Part print with two shaded views. Sizes in mm from the minimum x, y, z corner. A direction names the side the tool comes from. Give positions to 0.01 mm unless a question says otherwise; leave off trailing zeros. Write each loop counter-clockwise with the first axis right and the second up, starting at its lowest first coordinate (ties: lowest second). Pieces come first, ordered by that corner, then holes. Notation, with made-up numbers: M 88,-13 L 143,-13 A25 ccw 143,14 Z; hole C -25,-21 d2. An arc over 180 degrees is marked long. Return JSON: item names as keys, results as strings. Group by question number.
Q1. Pull direction Y, two halves, no side cores. Call the marked faces 3, 4 and 5: +Y half, -Y half, draft (parallel to the pull), parting line (faces both ways), or undercut.
Q2. Tool access for the marked faces 1 and 2: list every direction of +Z, -Z, +X, -X, +Y, -Y with a clear straight run to the whole face (end or side of a thin tool).
Q3. Wall check: probe 1 along Y at (x, z) = (6, 11) (1 decimal); probe 2 along Y at (x, z) = (9.5, 18.5) (1 decimal); probe 3 along Z at (x, y) = (16.5, 10.5). Give the ranges that are in metal, low to high.
Q4. Band-saw the part on A-A, the plane z = 16. Give the cut face in (x, y) (1 decimal).
Q5. Band-saw the part on C-C, the plane y = 11. Give the cut face in (x, z).
Q6. Flat gauge pins, fed straight in: pin 1 Ø0.9 at (x, z) = (17.52, 3.17) entering from +Y; pin 2 Ø1 at (x, y) = (11.5, 12) entering from -Z; pin 3 Ø1.5 at (x, y) = (19, 16) entering from -Z. Where does each tip first touch, or does it go through?
Q7. Band-saw the part on B-B, the plane x = 9. Give the cut face in (y, z) (1 decimal).
Q8. Band-saw the part on D-D, the plane x = 13. Give the cut face in (y, z) (1 decimal).
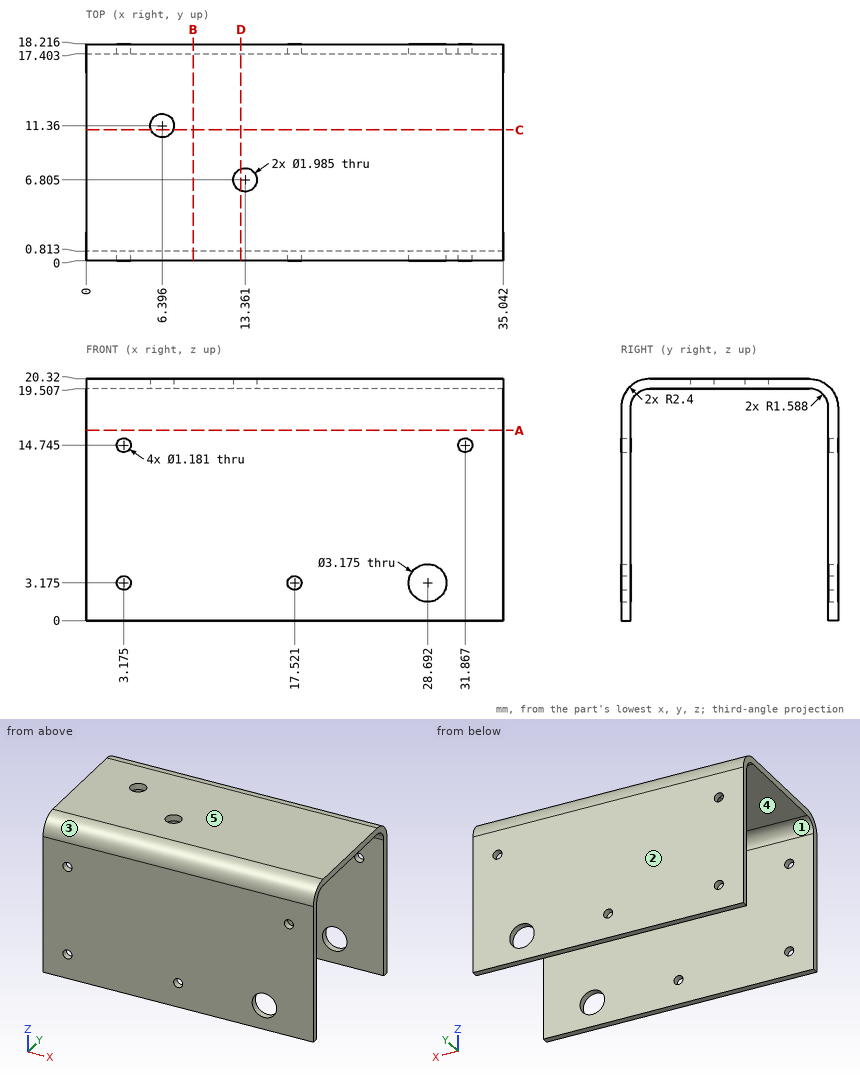
From the geometry:
{
 "1": {"face 3": "-Y half", "face 4": "undercut", "face 5": "draft"},
 "2": {"face 1": "-Z, +X, -X", "face 2": "+Z, -Z, +X, -X, +Y"},
 "3": {"probe 1": "y = 0 to 0.8, 17.4 to 18.2", "probe 2": "y = 0.1 to 0.9, 17.3 to 18.1", "probe 3": "z = 19.51 to 20.32"},
 "4": {"outline": "M 0,0 L 35,0 L 35,0.8 L 0,0.8 Z; M 0,17.4 L 35,17.4 L 35,18.2 L 0,18.2 Z"},
 "5": {"outline": "M 0,19.51 L 5.47,19.51 L 5.47,20.32 L 0,20.32 Z; M 7.32,19.51 L 35.04,19.51 L 35.04,20.32 L 7.32,20.32 Z"},
 "6": {"pin 1": "passes through", "pin 2": "stops at z = 19.51", "pin 3": "stops at z = 19.2"},
 "7": {"outline": "M 0,0 L 0.8,0 L 0.8,17.9 A1.6 cw 2.4,19.5 L 15.8,19.5 A1.6 cw 17.4,17.9 L 17.4,0 L 18.2,0 L 18.2,17.9 A2.4 ccw 15.8,20.3 L 2.4,20.3 A2.4 ccw 0,17.9 Z"},
 "8": {"outline": "M 0,0 L 0.8,0 L 0.8,17.9 A1.6 cw 2.4,19.5 L 5.9,19.5 L 5.9,20.3 L 2.4,20.3 A2.4 ccw 0,17.9 Z; M 7.7,19.5 L 15.8,19.5 A1.6 cw 17.4,17.9 L 17.4,0 L 18.2,0 L 18.2,17.9 A2.4 ccw 15.8,20.3 L 7.7,20.3 Z"}
}
